For this review, use the dimensioned drawing (mm, ordinates from the lowest corner) and the shaded views. A direction names the side the tool comes from. Give positions to 0.01 mm unless a question says otherwise; leave off trailing zeros. Order: outer loops, then holes, each group sorted by start corner. A loop starts at its lowest first (then second) coordinate and runs counter-clockwise, first axis right, second up. Notation, with made-up numbers: (-33.5, -10) - (24.5, -10) arc R18 cw to (24.5, 16) - close; hole circle Ø4 at (87, 77). An arc over 180 degrees is marked (long way). Use a Markdown table: item, result. Add a question column.
1) Wall thickness on L1, parallel to Z at x = 2.25, y = 1.75; L2, parallel to X at y = 3.5, z = 10; L3, parallel to Y at x = 2.5, z = 10.5: over which ranges is each line inside the solid? List them lowest first.
2) We need section C-C on z = 10.75. Write out the cut boundary in (x, y).
3) Machinability: for the marked faces 1 and 2, which of the approach directions +Z, -Z, +X, -X, +Y, -Y give a long, thin tool a straight path to every point of the face, cutting with its end or side? Answer none if there is none.
4) We need section D-D on x = 7. Write out the cut boundary in (y, z).
5) We need section A-A on y = 4. Write out the cut boundary in (x, z), then the cut area to 3 significant figures.
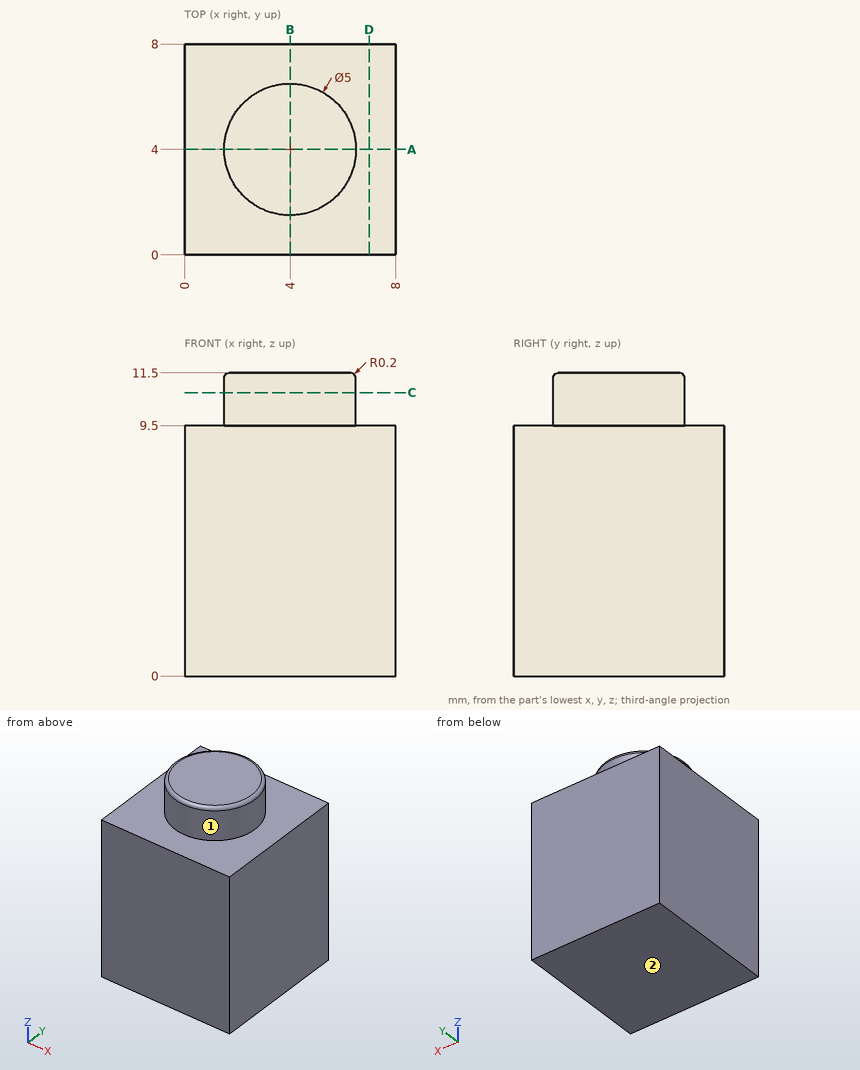
Checked values:
| question | item | result |
|---|---|---|
| 1 | L1 | 0 to 9.5 |
| 1 | L2 | 1.55 to 6.45 |
| 1 | L3 | 2 to 6 |
| 2 | outline | circle Ø5 at (4, 4) |
| 3 | face 1 | +Z |
| 3 | face 2 | -Z, +X, -X, +Y, -Y |
| 4 | outline | (0, 0) - (8, 0) - (8, 9.5) - (0, 9.5) - close |
| 5 | outline | (0, 0) - (8, 0) - (8, 9.5) - (6.5, 9.5) - (6.5, 11.3) arc R0.2 ccw to (6.3, 11.5) - (1.7, 11.5) arc R0.2 ccw to (1.5, 11.3) - (1.5, 9.5) - (0, 9.5) - close |
| 5 | area | 86.0 mm² |
